Geometry: see drawing. Coordinates: mm, zero at the bounding-box minimum. A direction names the side the tool comes from. Coordinates: 2 decimals unless noted, no trailing zeros. Loops run counter-clockwise (first coordinate to the right, second up) from the corner with the lowest first, then second, coordinate; pieces in that order, holes last. Notation, with made-up numbers: M 78,4 L 126,4 A14 cw 126,10 Z; hole C 79,26.25 d2. An arc over 180 degrees is marked long. One line per question, with ' | ' between items. Start each with the question number.
1. Section query D-D, the plane z = 13. Output: boundary loops of the cut face in (x, y), and give its area (3 significant figures).
2. Ray query, probe 1 along Y at (x, z) = (14, 19.5); probe 2 along Z at (x, y) = (20.75, 19); probe 3 along X at (y, z) = (23.5, 6.75). Return the intervals inside material, ascending.
3. Mould query, pull axis Y, two halves, no side actions, for the marked faces 3, 4, 5 and 6. Classes: pulls with the +Y half, pulls with the -Y half, needs draft (parallel to the pull), parting line crosses it, or undercut.
4. Section query B-B, the plane z = 15.5. Output: boundary loops of the cut face in (x, y).
5. Section query C-C, the plane y = 12. Output: boundary loops of the cut face in (x, z), and give its area (3 significant figures).
6. Section query A-A, the plane x = 14. Output: boundary loops of the cut face in (y, z).
7. Pin query (flat end, axial travel): P1, Ø5.5, axis at x = 20.5, y = 43.5, coming from the -Z side; P2, Ø4.5, axis at x = 20.5, z = 4.5, coming from the +Y side; P3, Ø2.5, axis at y = 42, z = 5.5, coming from the +X side. Return the tip coordinate at first contact, or that it passes through.
8. Access query for the marked faces 1 and 2. Directions: +Z, -Z, +X, -X, +Y, -Y. A direction counts if a zero-diameter tool reaches every point of the face in a straight line with its end or side. Return the directions, or none.
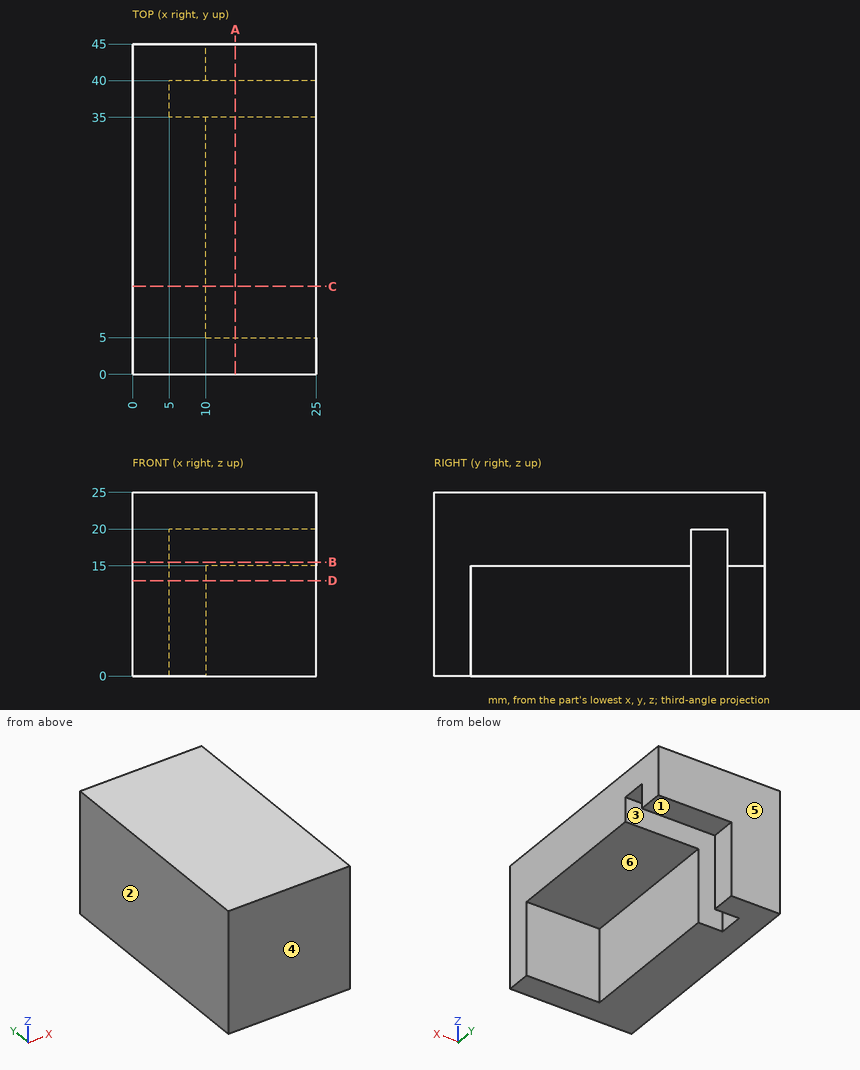
Taken from the geometry:
1) outline: M 0,0 L 25,0 L 25,5 L 10,5 L 10,35 L 5,35 L 5,40 L 10,40 L 10,45 L 0,45 Z | area: 500 mm^2
2) probe 1: 0 to 35, 40 to 45 | probe 2: 15 to 25 | probe 3: 0 to 10
3) face 3: undercut | face 4: pulls with the -Y half | face 5: pulls with the +Y half | face 6: needs draft
4) outline: M 0,0 L 25,0 L 25,35 L 5,35 L 5,40 L 25,40 L 25,45 L 0,45 Z
5) outline: M 0,0 L 10,0 L 10,15 L 25,15 L 25,25 L 0,25 Z | area: 400 mm^2
6) outline: M 0,0 L 5,0 L 5,15 L 35,15 L 35,20 L 40,20 L 40,15 L 45,15 L 45,25 L 0,25 Z
7) P1: z = 15 | P2: y = 5 | P3: x = 10
8) face 1: -Z, +X, +Y | face 2: +Z, -Z, -X, +Y, -Y
